Model file for the job. Use its own axes, mm. Round coordinates to 2 decimals unless told otherwise and drop trailing zeros. Loops run counter-clockwise (first coordinate to the right, second up) from the corner with the lowest first, then second, coordinate; pieces in that order, holes last. Notation, with made-up numbers: M -12,83.25 L 35,83.25 A25 ccw 35,118.25 Z; hole C 85.25,44 d7. An arc over 180 degrees is marked long. Use a Markdown table: item, result. Add a question column.
Q1. Pin check, flat tips, straight feed: pin 1 (1.5 mm diameter, centred on x = 9, z = 8.5, fed in from -Y); pin 2 (3 mm diameter, centred on y = 29.5, z = 4, fed in from -X); pin 3 (3 mm diameter, centred on y = 51.5, z = 1.5, fed in from -X); pin 4 (9 mm diameter, centred on x = -52.5, y = -42.5, fed in from +Z). Stop position of each tip, or through.
Q2. Mould opens along Y. For faces 1 (the face through (50.473, -40.641, 6.278)), 2 (the face through (-1, -16, 10)), 3 (the face through (-59.517, -45.636, 4.93)), 4 (the face through (-54.527, -40.641, 6.278)) say: +Y half, -Y half, draft (parallel to the pull), parting line (faces both ways), or undercut.
Q3. Cut at D-D (y = 42.5). Give the cut face in (x, z), plus the area to 3 significant figures.
Q4. Cut at A-A (y = 0). Give the cut face in (x, z), plus the area to 3 significant figures.
Q5. Probe line 1 (Y direction, x = -52.5, z = 7.5); line 2 (Y direction, x = 0, z = 2.5); line 3 (X direction, y = 42.5, z = 5). List the from-to ranges inside material, lowest first. Write a range as from..to.
Q6. Cut at C-C (z = 5). Give the cut face in (x, y).
from build123d import *

# Parameters (mm, degrees)
SKETCH1_R                                       = 75
SKETCH1_R_2                                     = 7.5
BOSS_EXTRUDE1_DEPTH                             = 10
SKETCH2_R                                       = 1.5
CUT_EXTRUDE1_DEPTH                              = 107.536378763
CSK_FOR_M5_FLAT_HEAD_MACHINE_SCREW1_D           = 5.5
CSK_FOR_M5_FLAT_HEAD_MACHINE_SCREW1_CSINK_D     = 10.4
CSK_FOR_M5_FLAT_HEAD_MACHINE_SCREW1_CSINK_ANGLE = 90


with BuildPart() as part:
    # Sketch1 → Boss-Extrude1 (new body)
    with BuildSketch(Plane(origin=(0, 0, 0), x_dir=(0, 1, 0), z_dir=(0, 0, 1))):
        with Locations(Location((0, 0, 0), (0, 0, 270))):
            Circle(SKETCH1_R)
        with Locations(Location((0, 0, 0), (0, 0, 270))):
            Circle(SKETCH1_R_2, mode=Mode.SUBTRACT)
    extrude(amount=BOSS_EXTRUDE1_DEPTH)

    # Sketch2 → Cut-Extrude1 (cut, through all)
    with BuildSketch(Plane.XY.offset(10)):
        with Locations((-52.5, 42.5)):
            Circle(SKETCH2_R)
        with Locations((52.5, 42.5)):
            Circle(SKETCH2_R)
        with Locations((52.5, -42.5)):
            Circle(SKETCH2_R)
        with Locations((-52.5, -42.5)):
            Circle(SKETCH2_R)
    extrude(amount=-CUT_EXTRUDE1_DEPTH, mode=Mode.SUBTRACT)

    # CSK for M5 Flat Head Machine Screw1 (through all)
    with Locations(Plane(origin=(-52.5, -42.5, 0), x_dir=(-1, 0, 0), z_dir=(0, 0, -1))):
        with Locations((0, 0), (-105, 0), (-105, 85), (0, 85)):
            CounterSinkHole(CSK_FOR_M5_FLAT_HEAD_MACHINE_SCREW1_D / 2, CSK_FOR_M5_FLAT_HEAD_MACHINE_SCREW1_CSINK_D / 2, counter_sink_angle=CSK_FOR_M5_FLAT_HEAD_MACHINE_SCREW1_CSINK_ANGLE)


solid = part.part
Checked values:
| question | item | result |
|---|---|---|
| 1 | pin 1 | stops at y = -74.54 |
| 1 | pin 2 | stops at x = -69.58 |
| 1 | pin 3 | stops at x = -55.9 |
| 1 | pin 4 | stops at z = 10 |
| 2 | face 1 | undercut |
| 2 | face 2 | draft |
| 2 | face 3 | parting line |
| 2 | face 4 | undercut |
| 3 | outline | M -61.8,0 L -57.7,0 L -55.25,2.45 L -55.25,10 L -61.8,10 Z; M -49.75,2.45 L -47.3,0 L 47.3,0 L 49.75,2.45 L 49.75,10 L -49.75,10 Z; M 55.25,2.45 L 57.7,0 L 61.8,0 L 61.8,10 L 55.25,10 Z |
| 3 | area | 1,110 mm^2 |
| 4 | outline | M -75,0 L -7.5,0 L -7.5,10 L -75,10 Z; M 7.5,0 L 75,0 L 75,10 L 7.5,10 Z |
| 4 | area | 1,350 mm^2 |
| 5 | line 1 | y = -53.56..-45.25, -39.75..39.75, 45.25..53.56 |
| 5 | line 2 | y = -75..-7.5, 7.5..75 |
| 5 | line 3 | x = -61.8..-55.25, -49.75..49.75, 55.25..61.8 |
| 6 | outline | C 0,0 d150; hole C -52.5,-42.5 d5.5; hole C -52.5,42.5 d5.5; hole C 0,0 d15; hole C 52.5,-42.5 d5.5; hole C 52.5,42.5 d5.5 |
